Design review of the part built by this model. Coordinates are the model's own, in mm. A direction names the side the tool comes from. Give positions to 0.01 mm unless a question says otherwise; leave off trailing zeros. Loops run counter-clockwise (first coordinate to the right, second up) from the corner with the lowest first, then second, coordinate; pieces in that order, holes last. Notation, with made-up numbers: (-19.75, -0.5) - (15.25, -0.5) arc R3 ccw to (15.25, 3.5) - close; hole circle Ø10 at (22, 3.5). An arc over 180 degrees is marked (long way). Write each question's results on one line, items separated by ' | '.
from build123d import *

# Parameters (mm, degrees)
SKETCH_1_R      = 1.25
EXTRUDE_1_DEPTH = 1.5


with BuildPart() as part:
    # 草图1 → 凸台-拉伸1 (new body)
    with BuildSketch(Plane.XY):
        with BuildLine():
            Line((61.485606927, 36.379045593), (55.661903622, 30.510449214))
            ThreePointArc((55.661903622, 30.510449214), (55.015327208, 29.534689328), (54.791375635, 28.385770659))
            Line((54.791375635, 28.385770659), (54.885447805, 3.885951263))
            Line((54.885447805, 3.885951263), (53.839506367, 3.049659841))
            Line((53.839506367, 3.049659841), (12.839808602, 2.892232945))
            Line((12.839808602, 2.892232945), (12.184344201, 27.942846038))
            ThreePointArc((12.184344201, 27.942846038), (11.926294769, 29.05242031), (11.284734435, 29.993773012))
            Line((11.284734435, 29.993773012), (6.389951155, 34.947075309))
            Line((6.389951155, 34.947075309), (5.188508902, 36.162881267))
            ThreePointArc((5.188508902, 36.162881267), (5.404097854, 41.328389075), (10.528570268, 40.643749035))
            Line((10.528570268, 40.643749035), (11.903832696, 38.663553725))
            Line((11.903832696, 38.663553725), (13.903817953, 38.671233086))
            Line((13.903817953, 38.671233086), (13.909577473, 37.171244144))
            Line((13.909577473, 37.171244144), (52.757056868, 37.320407148))
            Line((52.757056868, 37.320407148), (52.751297347, 38.820396091))
            Line((52.751297347, 38.820396091), (54.751282604, 38.828075452))
            Line((54.751282604, 38.828075452), (56.111289997, 40.818768719))
            ThreePointArc((56.111289997, 40.818768719), (61.230354838, 41.542747399), (61.485606927, 36.379045593))
        make_face()
        with Locations((59.00124888, 38.844398528)):
            Circle(SKETCH_1_R, mode=Mode.SUBTRACT)
        with Locations((7.653861631, 38.647239518)):
            Circle(SKETCH_1_R, mode=Mode.SUBTRACT)
        with BuildLine():
            Line((35.427528313, 24.013077802), (48.768603001, 34.305074976))
            Line((48.768603001, 34.305074976), (18.099515168, 34.187314613))
            Line((18.099515168, 34.187314613), (31.803272227, 23.982277822))
            ThreePointArc((31.803272227, 23.982277822), (33.620577188, 23.388506116), (35.427528313, 24.013077802))
        make_face(mode=Mode.SUBTRACT)
        with BuildLine():
            Line((40.287692252, 17.664023775), (51.865627723, 9.042062882))
            Line((51.865627723, 9.042062882), (51.780099927, 31.316616132))
            Line((51.780099927, 31.316616132), (40.250425641, 22.448057755))
            ThreePointArc((40.250425641, 22.448057755), (39.07959428, 20.046775087), (40.287692252, 17.664023775))
        make_face(mode=Mode.SUBTRACT)
        with BuildLine():
            Line((26.964065744, 22.301778302), (15.112244568, 31.102127061))
            Line((15.112244568, 31.102127061), (15.745126999, 8.829052268))
            Line((15.745126999, 8.829052268), (27.00804452, 17.517851185))
            ThreePointArc((27.00804452, 17.517851185), (28.175472686, 19.920749093), (26.964065744, 22.301778302))
        make_face(mode=Mode.SUBTRACT)
        with BuildLine():
            Line((48.877230949, 6.030566195), (35.448021091, 16.002175498))
            ThreePointArc((35.448021091, 16.002175498), (33.634102155, 16.593460395), (31.83047717, 15.971482382))
            Line((31.83047717, 15.971482382), (18.755497751, 5.914284289))
            Line((18.755497751, 5.914284289), (48.877230949, 6.030566195))
        make_face(mode=Mode.SUBTRACT)
    extrude(amount=EXTRUDE_1_DEPTH)


solid = part.part
(1) Insertion check: P1, Ø6, axis at x = 28, y = 8.5, coming from the -Z side; P2, Ø3, axis at x = 10.5, y = 10, coming from the +Z side. Each pin has a flat end and moves straight along its axis. Give the tip position at first contact, or say it passes through.
Answers below:
P1: z = 0 | P2: through
(2) Take a section at B-B on y = 25. Give the boundary of the cut face in (x, z), plus the area to 3 significant figures.
Answers below:
outline: (12.26, 0) - (15.29, 0) - (15.29, 1.5) - (12.26, 1.5) - close; (23.33, 0) - (30.44, 0) - (30.44, 1.5) - (23.33, 1.5) - close; (36.71, 0) - (43.57, 0) - (43.57, 1.5) - (36.71, 1.5) - close; (51.8, 0) - (54.8, 0) - (54.8, 1.5) - (51.8, 1.5) - close | area: 30.0 mm2
(3) Draft analysis for pull direction X (two halves, no side actions). For faces 1 (the flat face through (34, 23, 0)), 2 (the cylindrical face through (8.23, 37.54, 0.74)), 3 (the flat face through (58.615, 33.486, 0.74)), state which applies: pulls with the +X half, pulls with the -X half, needs draft (parallel to the pull), parting line crosses it, or undercut.
Answers below:
face 1: needs draft | face 2: undercut | face 3: pulls with the +X half
(4) Take a section at A-A on x = 43.5. Give the boundary of the cut face in (y, z), plus the area to 3 significant figures.
Answers below:
outline: (3.01, 0) - (6.01, 0) - (6.01, 1.5) - (3.01, 1.5) - close; (10.02, 0) - (15.27, 0) - (15.27, 1.5) - (10.02, 1.5) - close; (24.95, 0) - (30.24, 0) - (30.24, 1.5) - (24.95, 1.5) - close; (34.28, 0) - (37.28, 0) - (37.28, 1.5) - (34.28, 1.5) - close | area: 24.8 mm2
(5) Wall thickness on line 1 along Y through (x, z) = (47, 0.45); line 2 along X through (y, z) = (28, 0.9); line 3 along Y through (x, z) = (46, 0.2): over which ranges is each line inside the solid? List them lowest first. Write a range as from..to.
Answers below:
line 1: 3.02..6.02, 7.42..12.67, 27.64..32.94, 34.3..37.3 | line 2: 12.18..15.2, 19.29..26.41, 40.6..47.47, 51.79..54.79 | line 3: 3.02..6.02, 8.17..13.41, 26.87..32.17, 34.29..37.29
(6) Take a section at D-D on y = 19.5. Give the boundary of the cut face in (x, z).
Answers below:
outline: (12.41, 0) - (15.44, 0) - (15.44, 1.5) - (12.41, 1.5) - close; (28.15, 0) - (39.13, 0) - (39.13, 1.5) - (28.15, 1.5) - close; (51.83, 0) - (54.83, 0) - (54.83, 1.5) - (51.83, 1.5) - close
(7) Tool access review of faces 4 (the flat face through (55.42, 39.81, 0.74)), 5 (the flat face through (34, 23, 1.5)), 6 (the cylindrical face through (28.176, 19.882, 0.74)): name each direction out of +Z, -Z, +X, -X, +Y, -Y from which nothing blocks a thin tool from reaching the whole face with its end or side.
Answers below:
face 4: +Z, -Z, +Y | face 5: +Z, +X, -X, +Y, -Y | face 6: +Z, -Z
(8) Take a section at C-C on x = 37. Give the boundary of the cut face in (y, z) (3 decimals), plus the area to 3 significant figures.
Answers below:
outline: (2.985, 0) - (5.985, 0) - (5.985, 1.5) - (2.985, 1.5) - close; (14.85, 0) - (25.226, 0) - (25.226, 1.5) - (14.85, 1.5) - close; (34.26, 0) - (37.26, 0) - (37.26, 1.5) - (34.26, 1.5) - close | area: 24.6 mm2
